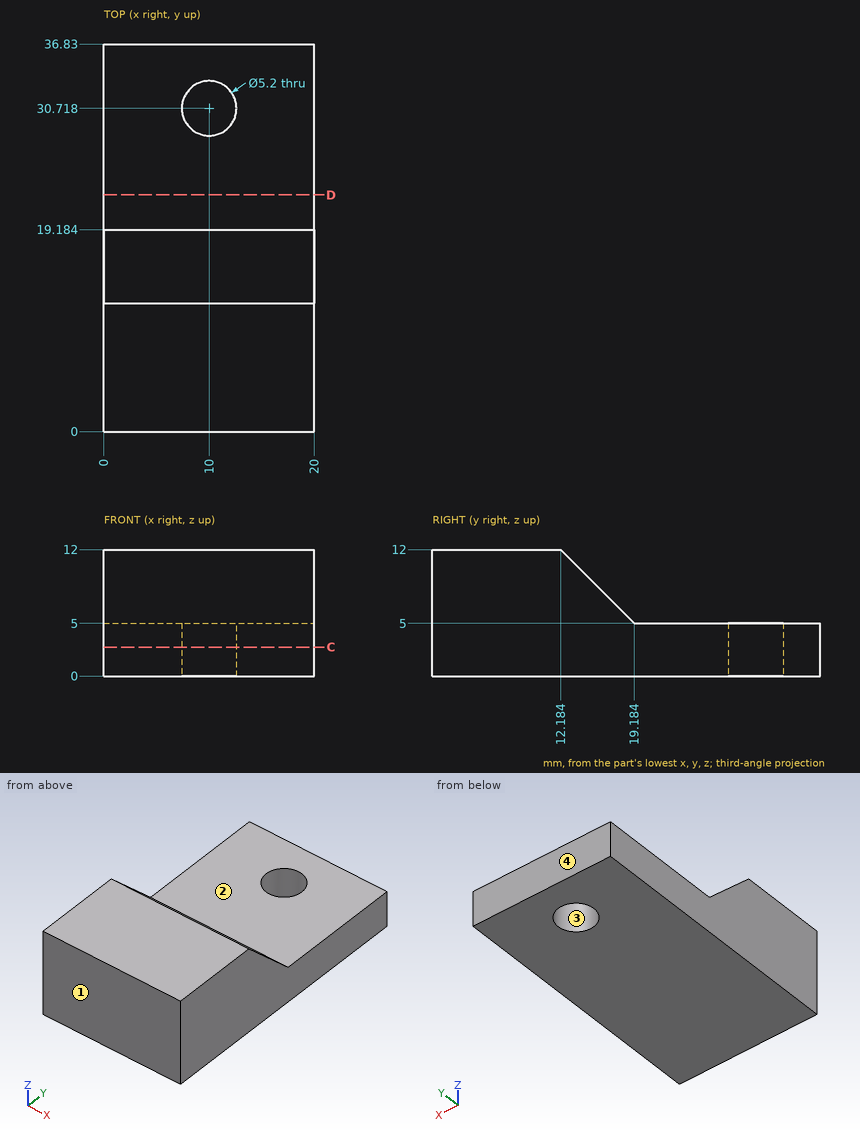
Design review of the part shown in the three views and the two pictorial views. Dimensions are in mm from the part's minimum x, y and z. Round coordinates to 2 decimals unless told otherwise and drop trailing zeros. Write each loop counter-clockwise with the first axis right and the second up, starting at its lowest first coordinate (ties: lowest second). Pieces come first, ordered by that corner, then holes.
Item 1: Clearance check with a flat-ended pin moving along its axis: pin 1 Ø5.5 at (x, y) = (10, 31) entering from +Z. State where the tip first meets the part, or that it passes through.
Item 2: The part is to be moulded in two halves that separate along Y. For the marked faces 1, 2, 3 and 4, say which applies: +Y half, -Y half, draft (parallel to the pull), parting line (faces both ways), or undercut.
Item 3: For probe 1 along Y at (x, z) = (10, 2.15); probe 2 along Z at (x, y) = (13.5, 20); probe 3 along Y at (x, z) = (11.25, 1), list the stretches that pass through material, from the lowest coordinate up.
Item 4: We need section C-C on z = 2.75. Write out the cut boundary in (x, y).
Item 5: We need section D-D on y = 22.5. Write out the cut boundary in (x, z), and give its area (3 significant figures).
Returned:
1. pin 1: stops at z = 5
2. face 1: -Y half
2. face 2: draft
2. face 3: undercut
2. face 4: +Y half
3. probe 1: y = 0 to 28.12, 33.32 to 36.83
3. probe 2: z = 0 to 5
3. probe 3: y = 0 to 28.44, 33 to 36.83
4. outline: (0, 0) - (20, 0) - (20, 36.83) - (0, 36.83) - close; hole circle Ø5.2 at (10, 30.72)
5. outline: (0, 0) - (20, 0) - (20, 5) - (0, 5) - close
5. area: 100 mm2
